```python
from build123d import *

# Parameters (mm, degrees)
SKETCH3_W                = 4
SKETCH3_H                = 2.5
BOSS_EXTRUDE1_DEPTH      = 2.5
SKETCH6_W                = 1.5
SKETCH6_H                = 0.5
SKETCH6_W_2              = 0.5
SKETCH6_H_2              = 1.5
BOSS_EXTRUDE2_DEPTH      = 0.25
BOSS_EXTRUDE2_DEPTH_BACK = 0.25


with BuildPart() as part:
    # Sketch3 → Boss-Extrude1 (new body)
    with BuildSketch(Plane.XY):
        Rectangle(SKETCH3_W, SKETCH3_H)
    extrude(amount=BOSS_EXTRUDE1_DEPTH)

    # Sketch6 → Boss-Extrude2 (add, two sides)
    with BuildSketch(Plane.XY.offset(1.25)) as boss_extrude2_sk:
        with Locations((2.75, 0)):
            Rectangle(SKETCH6_W, SKETCH6_H)
        with Locations((3.75, 0)):
            Rectangle(SKETCH6_W_2, SKETCH6_H)
        with Locations((3.75, -1)):
            Rectangle(SKETCH6_W_2, SKETCH6_H_2)
        with Locations((-2.75, 0)):
            Rectangle(SKETCH6_W, SKETCH6_H)
        with Locations((-3.75, 0)):
            Rectangle(SKETCH6_W_2, SKETCH6_H)
        with Locations((-3.75, -1)):
            Rectangle(SKETCH6_W_2, SKETCH6_H_2)
    extrude(amount=BOSS_EXTRUDE2_DEPTH)
    extrude(boss_extrude2_sk.sketch, amount=-BOSS_EXTRUDE2_DEPTH_BACK)


solid = part.part
```
The listing builds one solid part. Answer for the finished solid, in the listing's coordinates (mm). A direction names the side the tool comes from. Round coordinates to 2 decimals unless told otherwise and drop trailing zeros. Loops run counter-clockwise (first coordinate to the right, second up) from the corner with the lowest first, then second, coordinate; pieces in that order, holes last.
1) A cutting plane is placed at A-A on y = -1.4. Determine the outline of the cut face in (x, z).
Outcome:
outline: (-4, 1) - (-3.5, 1) - (-3.5, 1.5) - (-4, 1.5) - close; (3.5, 1) - (4, 1) - (4, 1.5) - (3.5, 1.5) - close
2) For faces 1 (the face through (3.7, -0.3, 1)), 2 (the face through (-3, 0, 1)), 3 (the face through (-3, 0, 1.5)), determine the directions among +Z, -Z, +X, -X, +Y, -Y from which every point of the face is accessible in a straight line to the end or side of a thin tool.
Outcome:
face 1: -Z, +X, +Y, -Y
face 2: -Z, -X, +Y, -Y
face 3: +Z, -X, +Y, -Y
3) A cutting plane is placed at D-D on y = -0.1. Determine the outline of the cut face in (x, z).
Outcome:
outline: (-4, 1) - (-2, 1) - (-2, 0) - (2, 0) - (2, 1) - (4, 1) - (4, 1.5) - (2, 1.5) - (2, 2.5) - (-2, 2.5) - (-2, 1.5) - (-4, 1.5) - close
4) A cutting plane is placed at B-B on y = -0.7. Determine the outline of the cut face in (x, z), plus the area to 3 significant figures.
Outcome:
outline: (-4, 1) - (-3.5, 1) - (-3.5, 1.5) - (-4, 1.5) - close; (-2, 0) - (2, 0) - (2, 2.5) - (-2, 2.5) - close; (3.5, 1) - (4, 1) - (4, 1.5) - (3.5, 1.5) - close
area: 10.5 mm2
5) Consider line 1 (Y direction, x = -0.75, z = 1.7); line 2 (X direction, y = -1.2, z = 0.2); line 3 (X direction, y = -1.4, z = 1.1). Determine where each line is inside the solid, lowest interval first.
Outcome:
line 1: y = -1.25 to 1.25
line 2: x = -2 to 2
line 3: x = -4 to -3.5, 3.5 to 4
6) Given P1, Ø0.8, axis at x = 1, z = 0.5, coming from the -Y side; P2, Ø0.6, axis at x = 2.5, y = -0.5, coming from the +Z side; P3, Ø0.6, axis at x = -3, z = 1.5, coming from the +Y side, each flat-ended and moving along its own axis, determine where each tip first touches the part or whether it passes through.
Outcome:
P1: stops at y = -1.25
P2: stops at z = 1.5
P3: stops at y = 0.25
7) A cutting plane is placed at C-C on z = 1.25. Determine the outline of the cut face in (x, y).
Outcome:
outline: (-4, -1.75) - (-3.5, -1.75) - (-3.5, -0.25) - (-2, -0.25) - (-2, -1.25) - (2, -1.25) - (2, -0.25) - (3.5, -0.25) - (3.5, -1.75) - (4, -1.75) - (4, 0.25) - (2, 0.25) - (2, 1.25) - (-2, 1.25) - (-2, 0.25) - (-4, 0.25) - close
